```python
from build123d import *

# Parameters (mm, degrees)
F2_DEPTH = 8


with BuildPart() as f2:
    # F1 (on Top) → F2 (new body)
    with BuildSketch(Plane.XY):
        Polygon((-0.07, -4.5), (-2, -3), (-2, -1), (0, -1), (0, 0), (-4, 0), (-4, -6), (-2, -6), align=None)
    extrude(amount=F2_DEPTH)

    # F3: F2 across plane


with BuildPart() as f2_1:
    add(f2.part)
    add(f2.part.mirror(Plane.YZ))

    # F4: F2 across plane


with BuildPart() as f2_2:
    add(f2_1.part)
    add(f2_1.part.mirror(Plane.XZ))


solid = f2_2.part
```
Could you check a few things on this model? Use its own coordinates, in mm. A direction names the side the tool comes from. Round coordinates to 2 decimals unless told otherwise and drop trailing zeros. Loops run counter-clockwise (first coordinate to the right, second up) from the corner with the lowest first, then second, coordinate; pieces in that order, holes last. Notation, with made-up numbers: M -38,81 L -19,81 A27 ccw -19,111 Z; hole C 71.5,22.5 d5. An arc over 180 degrees is marked long. Answer as CSV lines item,"result".
1) Which directions (+Z, -Z, +X, -X, +Y, -Y) give clear straight access to the entire face, cutting with the end or side of a thin tool? Please do faces 4 (the flat face through (-2, -2, 4)), 5 (the flat face through (1.05, 5.26, 3.94)), 6 (the flat face through (1.05, -5.26, 3.94)).
From the geometry:
face 4,"+Z, -Z"
face 5,"+Z, -Z, +Y"
face 6,"+Z, -Z, -Y"
2) Imagine slicing it at C-C on y = -5. List the corners of the cut face in (x, z) for me.
From the geometry:
outline,"M -4,0 L -0.71,0 L -0.71,8 L -4,8 Z; M 0.71,0 L 4,0 L 4,8 L 0.71,8 Z"
3) If I drill on probe 1 along X at (y, z) = (1.75, 6); probe 2 along Y at (x, z) = (-1.75, 6); probe 3 along Y at (x, z) = (0.5, 1), over which ranges is the centre line in solid material (lowest first)?
From the geometry:
probe 1,"-4 to -2, 2 to 4"
probe 2,"-5.81 to -3.19, -1 to 1, 3.19 to 5.81"
probe 3,"-4.83 to -4.17, -1 to 1, 4.17 to 4.83"
4) We'd pull the mould along X, two halves only. Please class faces 1 (the flat face through (-1.02, -3.76, 3.94)), 2 (the flat face through (-4, 0, 4)), 3 (the flat face through (-3, 6, 4)): released by +X, released by -X, zero draft, split by the parting line, or undercut.
From the geometry:
face 1,"undercut"
face 2,"released by -X"
face 3,"zero draft"
5) Imagine slicing it at A-A on y = -2.5. List the corners of the cut face in (x, z) for me, and give its area (3 significant figures).
From the geometry:
outline,"M -4,0 L -2,0 L -2,8 L -4,8 Z; M 2,0 L 4,0 L 4,8 L 2,8 Z"
area,"32.0 mm^2"
6) Imagine slicing it at B-B on z = 2.5. List the corners of the cut face in (x, y) for me.
From the geometry:
outline,"M -4,-6 L -2,-6 L -0.07,-4.5 L -2,-3 L -2,-1 L 2,-1 L 2,-3 L 0.07,-4.5 L 2,-6 L 4,-6 L 4,6 L 2,6 L 0.07,4.5 L 2,3 L 2,1 L -2,1 L -2,3 L -0.07,4.5 L -2,6 L -4,6 Z"
